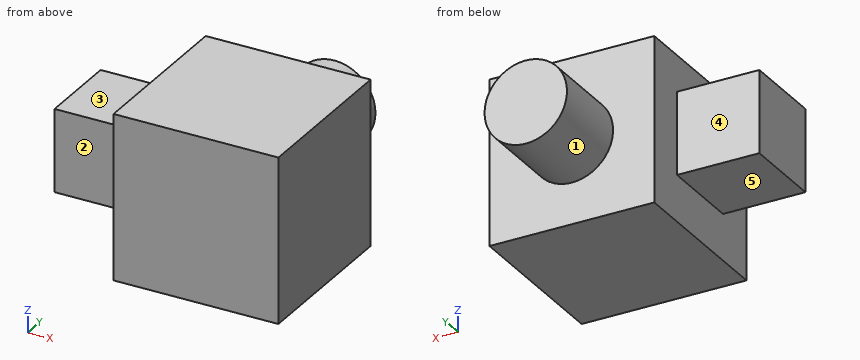
from build123d import *

# Parameters (mm, degrees)
F0_W     = 50.8
F0_H     = 50.8
F1_DEPTH = 50.8
F2_R     = 12.7
F3_DEPTH = 25.4
F4_W     = 25.4
F4_H     = 25.4
F5_DEPTH = 25.4


with BuildPart() as f1:
    # F0 (on Front) → F1 (new body)
    with BuildSketch(Plane.XZ):
        with Locations((19.548205, 25.4)):
            Rectangle(F0_W, F0_H)
    extrude(amount=F1_DEPTH)

    # F2 (on Front) → F3 (join)
    with BuildSketch(Plane.XZ):
        with Locations((19.548205, 25.4)):
            Circle(F2_R)
    extrude(amount=-F3_DEPTH)

    # F4 (on face) → F5 (join)
    with BuildSketch(Plane(origin=(-5.851795, 0, 0), x_dir=(0, -1, 0), z_dir=(-1, 0, 0))):
        with Locations((25.175295, 26.925846)):
            Rectangle(F4_W, F4_H)
    extrude(amount=F5_DEPTH)


solid = f1.part
CAD build for the part. Positions are in the model's coordinates, mm. Face numbers are marked on the shaded views. A direction names the side the tool comes from. Round coordinates to 2 decimals unless told otherwise and drop trailing zeros. Loops run counter-clockwise (first coordinate to the right, second up) from the corner with the lowest first, then second, coordinate; pieces in that order, holes last.
(1) Which spindle directions (+Z, -Z, +X, -X, +Y, -Y) get a long thin tool onto all of the face, cutting with end or side? Do the marked faces 1, 2, 3, 4 and 5. Say none if no direction does.
(2) Cut at D-D (x = -11). Give the cut face in (y, z).
(3) Drop flat-ended pins along their axis: pin 1 (8 mm diameter, centred on y = 3.5, z = 21, fed in from -X); pin 2 (8 mm diameter, centred on x = -16.5, y = -23, fed in from +Z); pin 3 (20.5 mm diameter, centred on x = -23, y = -20.5, fed in from -Z). Give the stop position or say it passes through.
(4) Wall check: line 1 along X through (y, z) = (-11.5, 8); line 2 along Y through (x, z) = (10, 44.5); line 3 along Z through (x, y) = (-26.5, -21.5). Give the ranges that are in metal, low to high.
(5) Cut at A-A (z = 25.4). Give the cut face in (x, y).
(6) Cut at B-B (x = 24). Give the cut face in (y, z).
(7) Cut at C-C (y = 1). Give the cut face in (x, z).
Findings below:
1. face 1: +Y
1. face 2: +Z, -Z, -X, -Y
1. face 3: +Z, -X, +Y, -Y
1. face 4: +Z, -Z, -X, +Y
1. face 5: -Z, -X, +Y, -Y
2. outline: (-37.88, 14.23) - (-12.48, 14.23) - (-12.48, 39.63) - (-37.88, 39.63) - close
3. pin 1: stops at x = -5.85
3. pin 2: stops at z = 39.63
3. pin 3: stops at z = 14.23
4. line 1: x = -5.85 to 44.95
4. line 2: y = -50.8 to 0
4. line 3: z = 14.23 to 39.63
5. outline: (-31.25, -37.88) - (-5.85, -37.88) - (-5.85, -50.8) - (44.95, -50.8) - (44.95, 0) - (32.25, 0) - (32.25, 25.4) - (6.85, 25.4) - (6.85, 0) - (-5.85, 0) - (-5.85, -12.48) - (-31.25, -12.48) - close
6. outline: (-50.8, 0) - (0, 0) - (0, 13.51) - (25.4, 13.51) - (25.4, 37.29) - (0, 37.29) - (0, 50.8) - (-50.8, 50.8) - close
7. outline: circle Ø25.4 at (19.55, 25.4)
